Geometry check sheet. Reference: drawing and pictorial views, mm from the part's lowest x, y, z. A direction names the side the tool comes from. Coordinates: 2 decimals unless noted, no trailing zeros. Write each loop counter-clockwise with the first axis right and the second up, starting at its lowest first coordinate (ties: lowest second). Pieces come first, ordered by that corner, then holes.
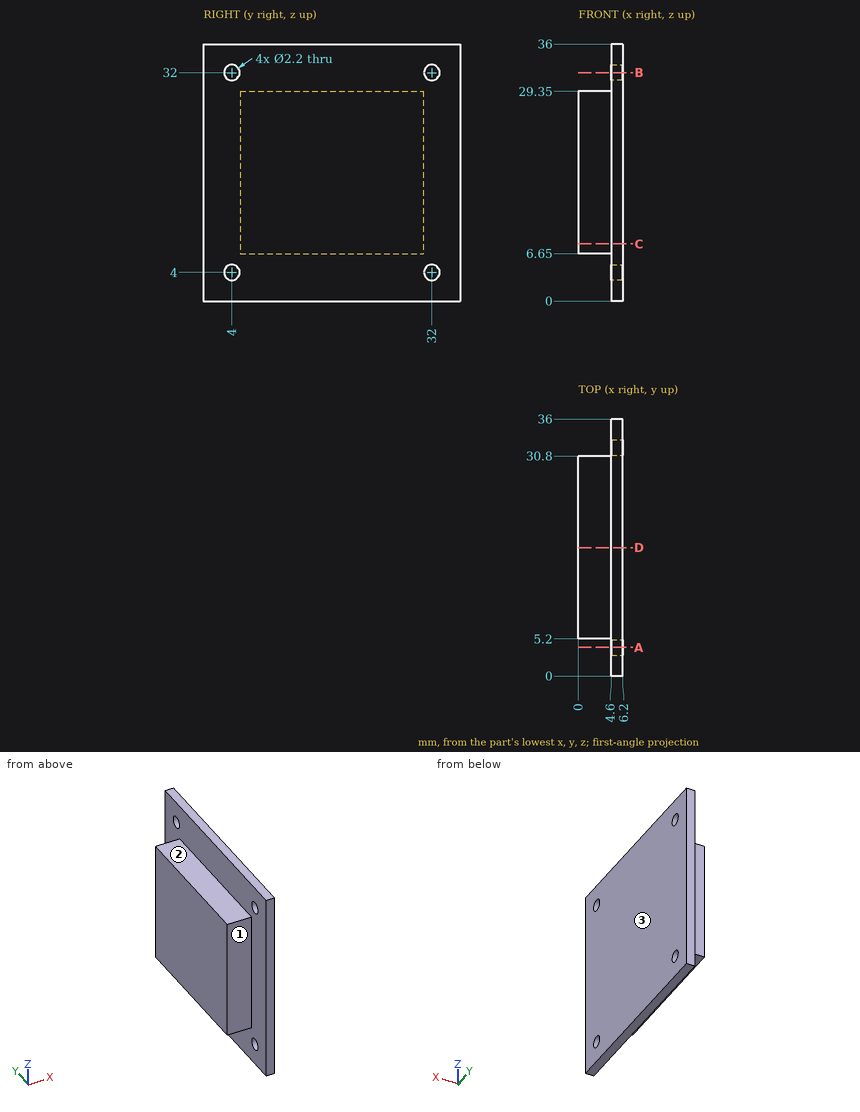
1. Sectioned sample at A-A, the plane y = 4. Record the boundary of the cut face in (x, z), and give its area (3 significant figures).
2. Gauge pin test, flat ends, axial feed: P1, Ø3, axis at x = 2, y = 26.5, coming from the +Z side; P2, Ø2.5, axis at x = 2.5, y = 14.5, coming from the -Z side; P3, Ø2.5, axis at x = 1, z = 14.5, coming from the +Y side; P4, Ø2, axis at y = 4, z = 32, coming from the +X side. Record the tip position at first contact, or that the pin passes through.
3. Sectioned sample at D-D, the plane y = 18. Record the boundary of the cut face in (x, z), and give its area (3 significant figures).
4. Sectioned sample at C-C, the plane z = 8. Record the boundary of the cut face in (x, y).
5. Tool access check on the marked faces 1, 2 and 3. Record the directions out of +Z, -Z, +X, -X, +Y, -Y that give a thin tool (end or side, any length) a straight path to the whole face; none if there is none.
6. Material ranges on L1, parallel to Z at x = 5, y = 32; L2, parallel to X at y = 31.5, z = 27, recorded low to high.
Outcome:
1. outline: (4.6, 0) - (6.2, 0) - (6.2, 2.9) - (4.6, 2.9) - close; (4.6, 5.1) - (6.2, 5.1) - (6.2, 30.9) - (4.6, 30.9) - close; (4.6, 33.1) - (6.2, 33.1) - (6.2, 36) - (4.6, 36) - close
1. area: 50.6 mm2
2. P1: stops at z = 29.35
2. P2: stops at z = 6.65
2. P3: stops at y = 30.8
2. P4: passes through
3. outline: (0, 6.65) - (4.6, 6.65) - (4.6, 0) - (6.2, 0) - (6.2, 36) - (4.6, 36) - (4.6, 29.35) - (0, 29.35) - close
3. area: 162 mm2
4. outline: (0, 5.2) - (4.6, 5.2) - (4.6, 0) - (6.2, 0) - (6.2, 36) - (4.6, 36) - (4.6, 30.8) - (0, 30.8) - close
5. face 1: +Z, -Z, -X, -Y
5. face 2: +Z, -X, +Y, -Y
5. face 3: +Z, -Z, +X, +Y, -Y
6. L1: z = 0 to 2.9, 5.1 to 30.9, 33.1 to 36
6. L2: x = 4.6 to 6.2
